Answer from the drawing. Dimensions are ordinates in mm from the lowest x, y and z of the part. A direction names the side the tool comes from. Round coordinates to 2 decimals unless told otherwise and drop trailing zeros. Write each loop counter-clockwise with the first axis right and the second up, starting at its lowest first coordinate (ties: lowest second). Pieces come first, ordered by that corner, then holes. Notation, with made-up numbers: (51, -30) -> (102, -30) arc R25 ccw to (102, -9) -> close; hole circle Ø3 at (20.5, 21). An arc over 180 degrees is marked (long way). Return JSON: item names as keys, results as strings. Group by question number.
(1) Given pin 1 (6 mm diameter, centred on y = 4.5, z = 38, fed in from +X); pin 2 (2.5 mm diameter, centred on x = 34.5, y = 4.5, fed in from +Z); pin 3 (10 mm diameter, centred on x = 17, z = 37, fed in from -Y); pin 4 (5 mm diameter, centred on x = 7.5, y = 7.5, fed in from -Z), each flat-ended and moving along its own axis, determine where each tip first touches the part or whether it passes through.
(2) Straight lines are drawn through the part: line 1 (X direction, y = 4.5, z = 49.5); line 2 (Y direction, x = 17.1, z = 22); line 3 (X direction, y = 5.75, z = 17.5). For each, find the intervals that lie inside material, in ascending order.
(3) A cutting plane is placed at C-C on y = 1.5. Give the vertices of the cut face in (x, z), then the cut area to 3 significant figures.
(4) A cutting plane is placed at B-B on y = 7.5. Give the vertices of the cut face in (x, z).
(5) For the marked faces 1, 2, 3, 4 and 5, determine the directions among +Z, -Z, +X, -X, +Y, -Y from which every point of the face is accessible in a straight line to the end or side of a thin tool.
(6) The mould has two halves that part along Z. Classify the marked faces 6, 7 and 8: released by +Z, released by -Z, zero draft, split by the parting line, or undercut.
(7) A cutting plane is placed at A-A on z = 3. Give the vertices of the cut face in (x, y), then the cut area to 3 significant figures.
(8) A cutting plane is placed at D-D on z = 16. Give the vertices of the cut face in (x, y).
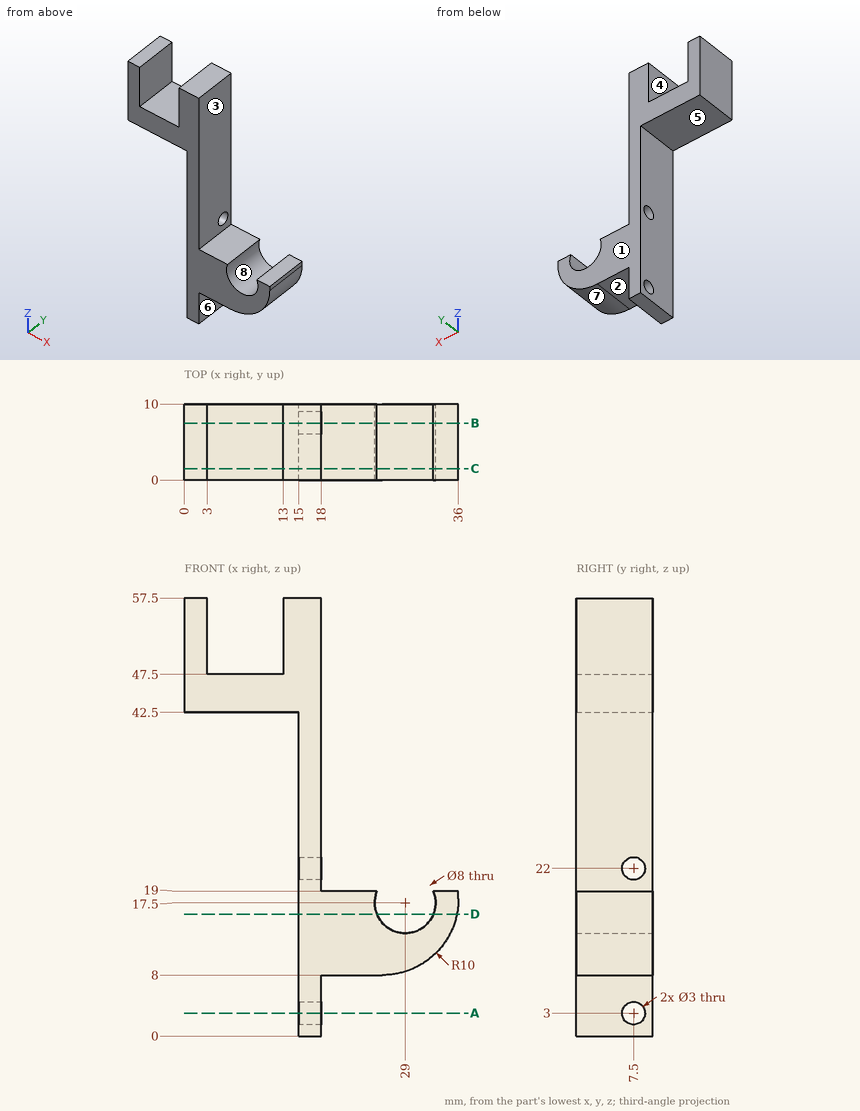
Checks:
{
 "1": {"pin 1": "stops at x = 18", "pin 2": "stops at z = 19", "pin 3": "stops at y = 0", "pin 4": "stops at z = 42.5"},
 "2": {"line 1": "x = 0 to 3, 13 to 18", "line 2": "y = 0 to 6, 9 to 10", "line 3": "x = 15 to 25, 33 to 35.99"},
 "3": {"outline": "(0, 42.5) -> (15, 42.5) -> (15, 0) -> (18, 0) -> (18, 8) -> (26, 8) arc R10 ccw to (36, 18) -> (36, 19) -> (32.71, 19) arc R4 cw (long way) to (25.29, 19) -> (18, 19) -> (18, 57.5) -> (13, 57.5) -> (13, 47.5) -> (3, 47.5) -> (3, 57.5) -> (0, 57.5) -> close", "area": "437 mm^2"},
 "4": {"outline": "(0, 42.5) -> (15, 42.5) -> (15, 23.5) -> (18, 23.5) -> (18, 57.5) -> (13, 57.5) -> (13, 47.5) -> (3, 47.5) -> (3, 57.5) -> (0, 57.5) -> close; (15, 0) -> (18, 0) -> (18, 1.5) -> (15, 1.5) -> close; (15, 4.5) -> (18, 4.5) -> (18, 8) -> (26, 8) arc R10 ccw to (36, 18) -> (36, 19) -> (32.71, 19) arc R4 cw (long way) to (25.29, 19) -> (18, 19) -> (18, 20.5) -> (15, 20.5) -> close"},
 "5": {"face 1": "+Z, -Z, +X, -X, +Y", "face 2": "-Z, +X, +Y, -Y", "face 3": "+Z, +X, +Y, -Y", "face 4": "+Z, +Y, -Y", "face 5": "-Z, -X, +Y, -Y"},
 "6": {"face 6": "zero draft", "face 7": "released by -Z", "face 8": "undercut"},
 "7": {"outline": "(15, 0) -> (18, 0) -> (18, 6) -> (15, 6) -> close; (15, 9) -> (18, 9) -> (18, 10) -> (15, 10) -> close", "area": "21.0 mm^2"},
 "8": {"outline": "(15, 0) -> (25.29, 0) -> (25.29, 10) -> (15, 10) -> close; (32.71, 0) -> (35.8, 0) -> (35.8, 10) -> (32.71, 10) -> close"}
}
